Geometry check sheet. Reference: the model listing, model coordinates, mm. Face numbers are marked on the shaded views. A direction names the side the tool comes from. Coordinates: 2 decimals unless noted, no trailing zeros. Write each loop counter-clockwise with the first axis right and the second up, starting at its lowest first coordinate (ties: lowest second). Pieces come first, ordered by that corner, then holes. Notation, with made-up numbers: (-8.5, -3) -> (46.5, -3) arc R19 cw to (46.5, 6) -> close; hole circle Ø5 at (2, -23.5). An arc over 180 degrees is marked (long way). One line per question, with ' | ' between items.
Autodesk Inventor part; units mm, degrees
ref_plane "YZ Plane" through (0, 0, 0) normal (1, 0, 0) x (0, 1, 0)
ref_plane "XZ Plane" through (0, 0, 0) normal (0, 1, 0) x (-1, 0, 0)
ref_plane "XY Plane" through (0, 0, 0) normal (0, 0, 1) x (1, 0, 0)
sketch "Sketch1" plane through (0, 0, 0) normal (0, 0, 1) x (1, 0, 0)
  line L0 (-14.1, -14.1) -> (14.1, -14.1)
  line L1 (14.1, -14.1) -> (14.1, 14.1)
  line L2 (14.1, 14.1) -> (-14.1, 14.1)
  line L3 (-14.1, 14.1) -> (-14.1, -14.1)
  line L4 (-14.1, -14.1) -> (14.1, 14.1) construction
  line L5 (14.1, -14.1) -> (-14.1, 14.1) construction
  point P0 (0, 0)
  dimension "d0" = 28.2
  dimension "d1" = 28.2
extrude "Extrusion1" add sketch "Sketch1" along normal blind 45
sketch "Sketch2" plane through (0, 0, 45) normal (0, 0, 1) x (1, 0, 0)
  circle A0 centre (0, 0) radius 11
  dimension "d4" = 22
extrude "Extrusion2" add sketch "Sketch2" along normal blind 2
sketch "Sketch3" plane through (0, 0, 47) normal (0, 0, 1) x (1, 0, 0)
  circle A0 centre (0, 0) radius 11
  circle A1 centre (0, 0) radius 2.5
  dimension "d7" = 5
extrude "Extrusion3" add sketch "Sketch3" along normal blind 18 contours A1
sketch "Sketch4" plane through (0, 0, 45) normal (0, 0, 1) x (1, 0, 0)
  circle A0 centre (0, 0) radius 11
  point P0 (-11.5, 11.5)
  point P1 (11.5, 11.5)
  point P2 (11.5, -11.5)
  point P3 (-11.5, -11.5)
  dimension "d10" = 11.5
  dimension "d11" = 11.5
  dimension "d12" = 11.5
  dimension "d13" = 11.5
  dimension "d14" = 11.5
  dimension "d15" = 11.5
  dimension "d16" = 11.5
  dimension "d17" = 11.5
hole "Hole1" at (-11.5, 11.5, 45) at (11.5, 11.5, 45) at (11.5, -11.5, 45) at (-11.5, -11.5, 45) direction (0, 0, -1) diameter 2.5 depth 4.5 tip angle 118
fillet "Fillet1" radius 2.5 4 edges at (-14.1, 14.1, 22.5) (14.1, 14.1, 22.5) (14.1, -14.1, 22.5) (-14.1, -14.1, 22.5)
fillet "Fillet2" radius 1 8 edges at (-13.3678, 13.3678, 0) (-14.1, 0, 0) (-13.3678, -13.3678, 0) (0, -14.1, 0) (13.3678, -13.3678, 0) (14.1, 0, 0) (13.3678, 13.3678, 0) (0, 14.1, 0)
properties part number "NEMA11"
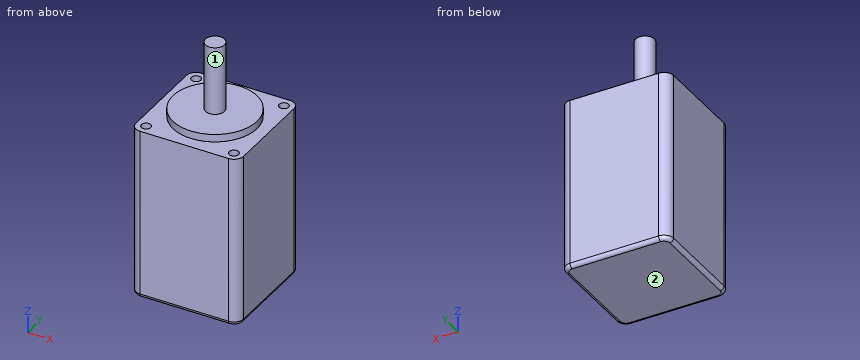
1. Go/stop test with flat-tipped pins: P1, Ø1.5, axis at x = 11.5, y = -11.5, coming from the +Z side; P2, Ø3, axis at x = 11.5, y = 11.5, coming from the +Z side; P3, Ø8.5, axis at x = 6.5, y = 2.5, coming from the +Z side; P4, Ø1, axis at x = -3.5, z = 58.5, coming from the +Y side. Record where each tip stops, or that it passes through.
Worked answers:
P1: z = 40.2 | P2: z = 45 | P3: z = 47 | P4: through
2. Tool access check on the marked faces 1 and 2. Record the directions out of +Z, -Z, +X, -X, +Y, -Y that give a thin tool (end or side, any length) a straight path to the whole face; none if there is none.
Worked answers:
face 1: +Z | face 2: -Z, +X, -X, +Y, -Y
3. Cross-section at C-C on z = 51. Record the boundary of the cut face in (x, y), and give its area (3 significant figures).
Worked answers:
outline: circle Ø5 at (0, 0) | area: 19.6 mm²
4. Material ranges on line 1 (X direction, y = -11.5, z = 42.4); line 2 (Z direction, x = -1.5, y = -4.75), recorded low to high. Write a range as from..to.
Worked answers:
line 1: -14.1..-12.75, -10.25..10.25, 12.75..14.1 | line 2: 0..47
5. Cross-section at B-B on x = -3.5. Record the boundary of the cut face in (y, z), and give its area (3 significant figures).
Worked answers:
outline: (-14.1, 1) arc R1 ccw to (-13.1, 0) -> (13.1, 0) arc R1 ccw to (14.1, 1) -> (14.1, 45) -> (10.43, 45) -> (10.43, 47) -> (-10.43, 47) -> (-10.43, 45) -> (-14.1, 45) -> close | area: 1,310 mm²
6. Cross-section at A-A on y = 0. Record the boundary of the cut face in (x, z).
Worked answers:
outline: (-14.1, 1) arc R1 ccw to (-13.1, 0) -> (13.1, 0) arc R1 ccw to (14.1, 1) -> (14.1, 45) -> (11, 45) -> (11, 47) -> (2.5, 47) -> (2.5, 65) -> (-2.5, 65) -> (-2.5, 47) -> (-11, 47) -> (-11, 45) -> (-14.1, 45) -> close
